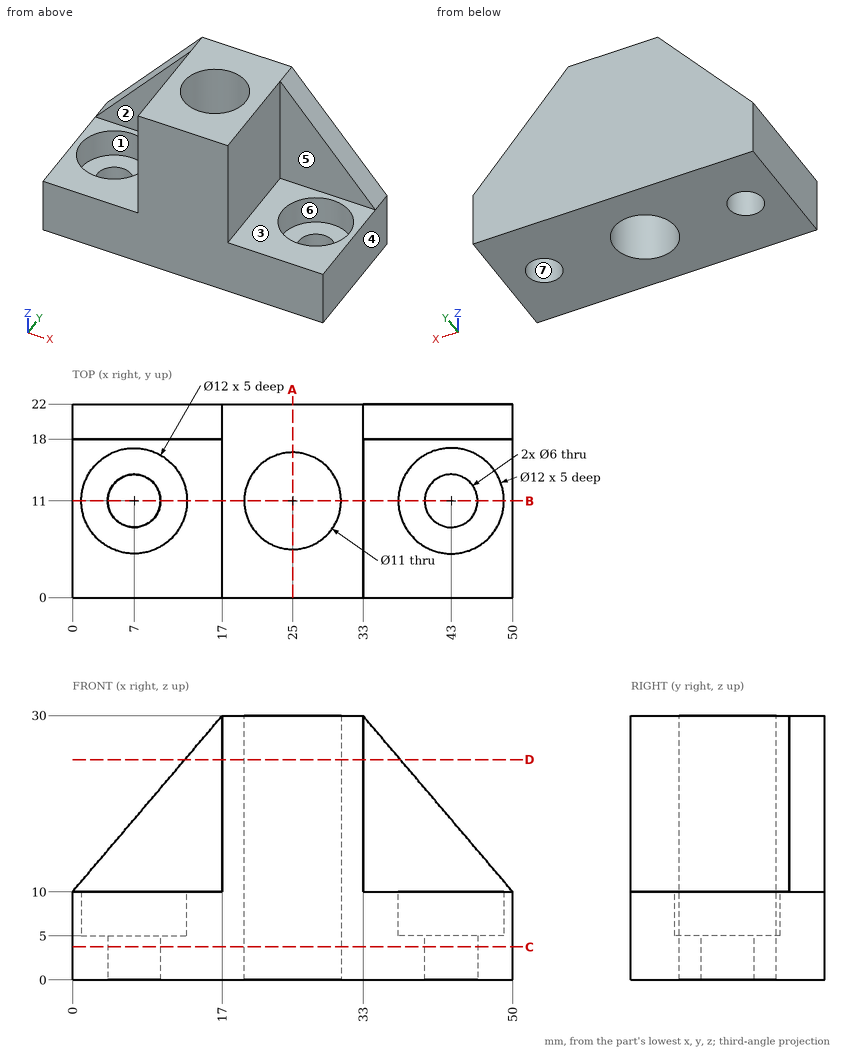
The figure shows three views and two pictorial views of one solid part (mm, origin at its lowest corner). Answer the questions. A direction names the side the tool comes from. Round coordinates to 2 decimals unless told otherwise and drop trailing zeros. Loops run counter-clockwise (first coordinate to the right, second up) from the corner with the lowest first, then second, coordinate; pieces in that order, holes last. Notation, with made-up numbers: (80.5, 89.25) - (95.5, 89.25) arc R35 cw to (95.5, 121.25) - close; hole circle Ø8 at (48.25, 6). An arc over 180 degrees is marked (long way). Use one line per item in the form item = value. Start each with the question number.
(1) Find section A-A on x = 25. Determine the outline of the cut face in (y, z).
(2) Find section B-B on y = 11. Determine the outline of the cut face in (x, z).
(3) Consider line 1 (Y direction, x = 7, z = 3.1); line 2 (Y direction, x = 25, z = 17); line 3 (X direction, y = 4.25, z = 11). Determine where each line is inside the solid, lowest interval first.
(4) Determine the mould class of the marked faces 4, 5, 6 and 7 for opening direction Y: +Y half, -Y half, draft (parallel to the pull), parting line (faces both ways), or undercut.
(5) Find section C-C on z = 3.75. Determine the outline of the cut face in (x, y), and give its area (3 significant figures).
(6) Flat-ended cylindrical pins translate along their axes: P1, Ø9.5, axis at x = 44, y = 9, coming from the +Z side; P2, Ø10, axis at y = 12.5, z = 26, coming from the -X side; P3, Ø5, axis at x = 38.5, z = 20, coming from the -Y side. Find the tip coordinate at first contact, or state that the pin passes through.
(7) Which of the six approach directions +Z, -Z, +X, -X, +Y, -Y give full straight-line access (tool end or side, diameter ignored) to the marked faces 1, 2 and 3?
(8) Find section D-D on z = 25. Determine the outline of the cut face in (x, y).
Answer list:
q1.outline = (0, 0) - (5.5, 0) - (5.5, 30) - (0, 30) - close; (16.5, 0) - (22, 0) - (22, 30) - (16.5, 30) - close
q2.outline = (0, 0) - (4, 0) - (4, 5) - (1, 5) - (1, 10) - (0, 10) - close; (10, 0) - (19.5, 0) - (19.5, 30) - (17, 30) - (17, 10) - (13, 10) - (13, 5) - (10, 5) - close; (30.5, 0) - (40, 0) - (40, 5) - (37, 5) - (37, 10) - (33, 10) - (33, 30) - (30.5, 30) - close; (46, 0) - (50, 0) - (50, 10) - (49, 10) - (49, 5) - (46, 5) - close
q3.line_1 = 0 to 8, 14 to 22
q3.line_2 = 0 to 5.5, 16.5 to 22
q3.line_3 = 17 to 33
q4.face_4 = draft
q4.face_5 = -Y half
q4.face_6 = undercut
q4.face_7 = undercut
q5.outline = (0, 0) - (50, 0) - (50, 22) - (0, 22) - close; hole circle Ø6 at (7, 11); hole circle Ø11 at (25, 11); hole circle Ø6 at (43, 11)
q5.area = 948 mm^2
q6.P1 = 10
q6.P2 = 17
q6.P3 = 18
q7.face_1 = +Z
q7.face_2 = +Z, -X, -Y
q7.face_3 = +Z, +X, -Y
q8.outline = (12.75, 18) - (17, 18) - (17, 0) - (33, 0) - (33, 18) - (37.25, 18) - (37.25, 22) - (12.75, 22) - close; hole circle Ø11 at (25, 11)
